The figure shows three views and two pictorial views of one solid part (mm, origin at its lowest corner). Answer the questions. Give positions to 0.01 mm unless a question says otherwise; leave off trailing zeros. Loops run counter-clockwise (first coordinate to the right, second up) from the corner with the lowest first, then second, coordinate; pieces in that order, holes last. Notation, with made-up numbers: (-39, 24) - (-5, 24) arc R34 ccw to (-5, 62) - close; hole circle Ø3 at (-4.5, -33). An arc over 180 degrees is marked (long way). One line per question, with ' | ' between items.
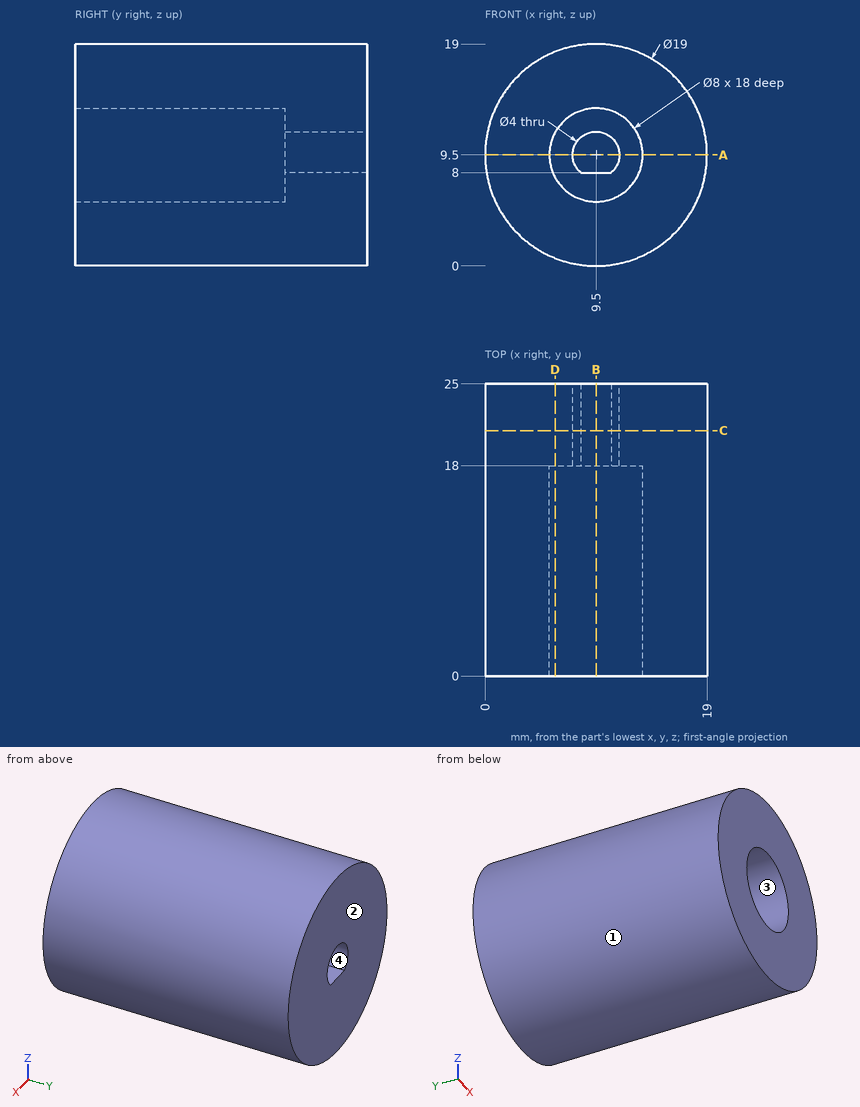
1. Find section C-C on y = 21. Write down the section's boundary in (x, z).
Evaluation:
outline: circle Ø19 at (9.5, 9.5); hole (8.18, 8) - (10.82, 8) arc R2 ccw (long way) to start
2. Flat-ended cylindrical pins translate along their axes: pin 1 (3 mm diameter, centred on y = 10, z = 13.5, fed in from +X); pin 2 (3 mm diameter, centred on y = 17.5, z = 16.5, fed in from -X); pin 3 (1 mm diameter, centred on x = 7, y = 21.5, fed in from +Z). Find the tip coordinate at first contact, or state that the pin passes through.
Evaluation:
pin 1: x = 18.67 | pin 2: x = 1.75 | pin 3: z = 18.79
3. Determine the mould class of the marked faces 1, 2, 3 and 4 for opening direction X: +X half, -X half, draft (parallel to the pull), parting line (faces both ways), or undercut.
Evaluation:
face 1: parting line | face 2: draft | face 3: undercut | face 4: undercut
4. Consider L1, parallel to Z at x = 9.5, y = 22; L2, parallel to X at y = 10, z = 9.5; L3, parallel to X at y = 22.75, z = 9.5. Determine where each line is inside the solid, lowest interval first.
Evaluation:
L1: 0 to 8, 11.5 to 19 | L2: 0 to 5.5, 13.5 to 19 | L3: 0 to 7.5, 11.5 to 19
5. Find section A-A on z = 9.5. Write down the section's boundary in (x, y).
Evaluation:
outline: (0, 0) - (5.5, 0) - (5.5, 18) - (7.5, 18) - (7.5, 25) - (0, 25) - close; (11.5, 18) - (13.5, 18) - (13.5, 0) - (19, 0) - (19, 25) - (11.5, 25) - close
6. Find section D-D on x = 6. Write down the section's boundary in (y, z), then the cut area to 3 significant figures.
Evaluation:
outline: (0, 0.67) - (25, 0.67) - (25, 18.33) - (0, 18.33) - (0, 11.44) - (18, 11.44) - (18, 7.56) - (0, 7.56) - close | area: 372 mm2
7. Find section B-B on x = 9.5. Write down the section's boundary in (y, z).
Evaluation:
outline: (0, 0) - (25, 0) - (25, 8) - (18, 8) - (18, 5.5) - (0, 5.5) - close; (0, 13.5) - (18, 13.5) - (18, 11.5) - (25, 11.5) - (25, 19) - (0, 19) - close
